For this review, take the finished solid that the model builds, in its own axes (mm). A direction names the side the tool comes from. Give positions to 0.01 mm unless a question says otherwise; leave off trailing zeros. Write each loop counter-clockwise with the first axis right and the second up, starting at its lowest first coordinate (ties: lowest second). Pieces come first, ordered by that corner, then holes. Notation, with made-up numbers: M 66.25,-23.5 L 95.25,-23.5 A21 ccw 95.25,3.5 Z; hole C 54,-30 d9. An arc over 180 degrees is marked long. Write item = value, one per line.
Autodesk Inventor part; units mm, degrees
ref_plane "Work Plane1" through (-15, 0, -27.5) normal (-1, 0, 0) x (0, -1, 0)
ref_plane "YZ Plane" through (0, 0, 0) normal (1, 0, 0) x (0, 1, 0)
ref_plane "XZ Plane" through (0, 0, 0) normal (0, 1, 0) x (-1, 0, 0)
sketch "Sketch1" plane through (0, 0, 0) normal (0, 1, 0) x (-1, 0, 0)
  line L0 (0, 0) -> (-25, 0)
  line L1 (-25, 0) -> (-25, -10)
  line L2 (-25, -10) -> (-15, -10)
  line L3 (-15, -10) -> (-15, -45)
  line L4 (-15, -45) -> (0, -45)
  line L5 (0, 0) -> (0, -45)
  dimension "d3" = 25
  dimension "d4" = 10
  dimension "d5" = 10
  dimension "d6" = 35
  dimension "d7" = 15
revolve "Revolution1" add sketch "Sketch1" angle 360 about axis through (0, 0, 0) along (0, 0, -1)
sketch "Sketch2" plane through (0, 0, 0) normal (0, 0, 1) x (1, 0, 0)
  line L0 (0, 0) -> (30.242, 0) construction
  line L1 (0, 0.5707) -> (22.435, 0.5707) construction
  circle A0 centre (9.7519, 17.4614) radius 2.25
  circle A1 centre (19.998, 0.2854) radius 2.25
  circle A2 centre (10.2461, -17.1761) radius 2.25
  circle A3 centre (-9.7519, -17.4614) radius 2.25
  circle A4 centre (-19.998, -0.2854) radius 2.25
  circle A5 centre (-10.2461, 17.1761) radius 2.25
  dimension "d12" = 4.5
  dimension "d15" = 360
extrude "Extrusion1" cut sketch "Sketch2" against normal through all
sketch "Sketch3" plane through (0, 0, 0) normal (0, 0, 1) x (1, 0, 0)
  circle A0 centre (0, 0) radius 5.5
  dimension "d19" = 11
extrude "Extrusion2" cut sketch "Sketch3" against normal through all
thread "Thread1"
sketch "Sketch4" plane through (0, 0, 0) normal (0, 0, 1) x (1, 0, 0)
  circle A0 centre (0, 0) radius 25
  line L0 (-17, 0) -> (-17, 18.3303)
  line L1 (-17, 0) -> (-17, -18.3303)
extrude "Extrusion3" cut sketch "Sketch4" against normal blind 15 contours L0 L1 A0 picked at (-18.2676, -10.7318)
ref_plane "Work Plane1" through (-15, 0, -27.5) normal (-1, 0, 0) x (0, -1, 0)
sketch "Sketch5" plane through (-15, 0, -27.5) normal (-1, 0, 0) x (0, -1, 0)
  line L0 (1.9646, 17.5) -> (-2.5354, 17.5)
  line L1 (15, -17.5) -> (-15, -17.5)
  line L2 (0, -11.5) -> (-5, -11.5)
  line L3 (-5.5, 27.5) -> (-5.5, -17.5)
  line L4 (-5, -11.5) -> (-5, 17.5)
  line L5 (15, 17.5) -> (-15, 17.5)
  line L6 (0, -11.5) -> (5, -11.5)
  line L7 (5, -11.5) -> (5, 17.5)
  line L8 (5, 17.5) -> (-5, 17.5)
  point P0 (0, 27.5)
extrude "Extrusion4" cut sketch "Sketch5" against normal blind 1
sketch "Sketch9" plane through (0, 0, -10) normal (0, 0, -1) x (-1, 0, 0)
  line L0 (14, 5) -> (14, -5)
  line L1 (14, 0) -> (22, 0)
  line L2 (22, 0) -> (22, -11.8743)
  line L3 (22, -11.8743) -> (22, 11.8743)
  arc A0 (22, 11.8743) -> (17.2515, 18.0938) centre (0, 0) ccw
  line L4 (17, -18.3303) -> (17, 18.3303)
  line L5 (17, 18.3303) -> (17, -18.3303)
  line L6 (17, 18.3303) -> (17, -18.3303)
  arc A1 (17, -18.3303) -> (22, -11.8743) centre (0, 0) ccw
  arc A2 (22, 11.8743) -> (17, 18.3303) centre (0, 0) ccw
  arc A3 (14.1421, 5) -> (14.1421, -5) centre (0, 0) ccw
  dimension "d59" = 8
extrude "Extrusion5" add sketch "Sketch9" against normal blind 10
sketch "Sketch20" plane through (-14, 0, -27.5) normal (-1, 0, 0) x (0, 0, 1)
  line L0 (17.5, -11.8743) -> (17.5, 11.8743)
  circle A0 centre (11.5, 9.25) radius 3.75
  line L1 (-17.5, -15) -> (-17.5, 15)
  line L2 (11.5, 9.25) -> (-3.7889, -9.25)
  circle A1 centre (-3.7889, -9.25) radius 3.75
  point P0 (27.5, 0)
  dimension "d85" = 7.5
  dimension "d87" = 24
  dimension "d88" = 7.5
extrude "Extrusion8" cut sketch "Sketch20" against normal blind 4.75
sketch "Sketch21" plane through (-22, -11.8743, -10) normal (0, 0, -1) x (-1, 0, 0)
  point P0 (-22, 11.8743)
sketch "Sketch22" plane through (-22, -11.8743, -10) normal (0, 0, -1) x (-1, 0, 0)
  point P0 (-22, 11.8743)
properties part number "nut"
1. Machinability: for faces 4 (the face through (-1.19, -5.37, -22.18)), 5 (the face through (-9.25, -9, -31)), 6 (the face through (13.856, 5.745, -27.745)), which of the approach directions +Z, -Z, +X, -X, +Y, -Y give a long, thin tool a straight path to every point of the face, cutting with its end or side? Answer none if there is none.
Responses:
face_4 = +Z, -Z
face_5 = -X
face_6 = -Z
2. We need section A-A, the plane x = 20.5. Write out the cut boundary in (y, z), then the cut area to 3 significant figures.
Responses:
outline = M -14.31,-10 L -1.91,-10 L -1.91,0 L -14.31,0 Z; M 2.48,-10 L 14.31,-10 L 14.31,0 L 2.48,0 Z
area = 242 mm2
3. Insertion check: P1, Ø4, axis at y = 5, z = -11, coming from the -X side; P2, Ø6, axis at x = 20, y = 0.29, coming from the -Z side; P3, Ø7, axis at y = -9.25, z = -31.29, coming from the +X side; P4, Ø3, axis at y = -1.5, z = -27, coming from the -X side. Each pin has a flat end and moves straight along its axis. Give the tip position at first contact, or say it passes through.
Responses:
P1 = -22
P2 = -10
P3 = 13.85
P4 = -14
4. We need section D-D, the plane y = 9.25. Write out the cut boundary in (x, z), then the cut area to 3 significant figures.
Responses:
outline = M -22,-10 L -11.81,-10 L -11.81,-12.25 L -9.25,-12.25 L -9.25,-19.75 L -11.81,-19.75 L -11.81,-45 L 11.81,-45 L 11.81,-10 L 23.23,-10 L 23.23,0 L -22,0 Z
area = 1,260 mm2
5. For line 1 along Y through (x, z) = (0, -31); line 2 along Y through (x, z) = (0, -9); line 3 along Z through (x, y) = (16, 4), list the stretches that pass through material, from the lowest coordinate up. Write a range as from..to.
Responses:
line_1 = -15..-5.5, 5.5..15
line_2 = -25..-5.5, 5.5..25
line_3 = -10..0
6. The part is to be moulded in two halves that separate along X. For faces 1 (the face through (18.34, 1.806, -4.93)), 2 (the face through (-22, 0, -5)), 3 (the face through (0, 6, -45)), say which applies: +X half, -X half, draft (parallel to the pull), parting line (faces both ways), or undercut.
Responses:
face_1 = undercut
face_2 = -X half
face_3 = draft
7. We need section C-C, the plane x = 1. Write out the cut boundary in (y, z).
Responses:
outline = M -24.98,-10 L -14.97,-10 L -14.97,-45 L -5.41,-45 L -5.41,0 L -24.98,0 Z; M 5.41,-45 L 14.97,-45 L 14.97,-10 L 24.98,-10 L 24.98,0 L 5.41,0 Z
8. We need section B-B, the plane z = -16. Write out the cut boundary in (x, y).
Responses:
outline = M -14.14,-5 A15 ccw long -9.25,11.81 L -9.25,5.5 L -13.96,5.5 A15 ccw -14.14,5 L -14,5 L -14,-5 Z; hole C 0,0 d11
